Part model, mm, in its own coordinate system. Face numbers are marked on the shaded views. A direction names the side the tool comes from. Coordinates: 2 decimals unless noted, no trailing zeros. Write each loop counter-clockwise with the first axis right and the second up, starting at its lowest first coordinate (ties: lowest second). Pieces come first, ordered by that corner, then holes. Notation, with made-up numbers: (78, 10) -> (83, 10) arc R3 ccw to (83, 15) -> close; hole circle Ø5 at (88.5, 36). An arc over 180 degrees is marked (long way). Write item = value, one per line. Start each with the question number.
Q1. Band-saw the part on C-C, the plane y = 26.5. List the corners of the cut face in (x, z), plus the area to 3 significant figures.
Q2. Band-saw the part on A-A, the plane z = 21. List the corners of the cut face in (x, y), plus the area to 3 significant figures.
Q3. Probe line 1 (Z direction, x = 35.5, y = 18); line 2 (X direction, y = 26, z = 22); line 3 (Y direction, x = 20, z = 18). List the from-to ranges inside material, lowest first.
Q4. Band-saw the part on B-B, the plane x = 14. List the corners of the cut face in (y, z), plus the area to 3 significant figures.
Q5. Pull direction X, two halves, no side cores. Call the marked faces 3, 4, 5 and 6: released by +X, released by -X, zero draft, split by the parting line, or undercut.
Q6. Band-saw the part on D-D, the plane x = 4. List the corners of the cut face in (y, z).
Q7. Pin check, flat tips, straight feed: P1, Ø5, axis at x = 16.5, y = 18, coming from the +Z side; P2, Ø3, axis at x = 37, z = 17.5, coming from the -Y side. Stop position of each tip, or through.
Q8. Tool access for the marked faces 1 and 2: list every direction of +Z, -Z, +X, -X, +Y, -Y with a clear straight run to the whole face (end or side of a thin tool).
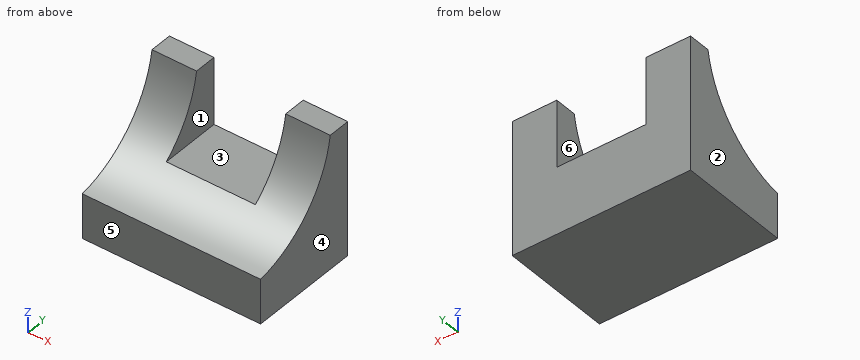
from build123d import *

# Parameters (mm, degrees)
F0_W     = 50.8
F0_H     = 12.7
F1_DEPTH = 31.75
F3_DEPTH = 6.35
F5_DEPTH = 25.4
F7_DEPTH = 50.8
F8_DEPTH = 25.4


with BuildPart() as f1:
    # F0 (on Front) → F1 (new body)
    with BuildSketch(Plane.XZ):
        with Locations((25.4, 6.35)):
            Rectangle(F0_W, F0_H)
    extrude(amount=-F1_DEPTH)

    # F2 (on face) → F3 (join)
    with BuildSketch(Plane(origin=(0, 31.75, 0), x_dir=(-1, 0, 0), z_dir=(0, 1, 0))):
        Polygon((-50.8, 38.1), (-50.8, 12.7), (0, 12.7), (0, 38.1), (-12.7, 38.1), (-12.7, 19.05), (-38.1, 19.05), (-38.1, 38.1), align=None)
    extrude(amount=-F3_DEPTH)

    # F4 (on face) → F5 (join)
    with BuildSketch(Plane.XY.offset(38.1)):
        Polygon((50.8, 0), (50.8, 25.4), (38.1, 25.4), (0, 25.4), (0, 0), align=None)
    extrude(amount=-F5_DEPTH)

    # F6 (on face) → F7 (cut)
    with BuildSketch(Plane.YZ.offset(50.8)):
        with BuildLine():
            Line((0, 38.1), (0, 12.7))
            ThreePointArc((0, 12.7), (16.8424565007, 21.2575434993), (25.4, 38.1))
            Line((25.4, 38.1), (0, 38.1))
        make_face()
    extrude(amount=-F7_DEPTH, mode=Mode.SUBTRACT)

    # F8 (cut): a face of the model
    f8_faces = [f1.faces().sort_by_distance(p)[0] for p in [
        (25.4, 25.4, 28.575),
    ]]
    extrude(f8_faces, amount=-F8_DEPTH, mode=Mode.SUBTRACT)


solid = f1.part
Ans:
q1.outline = (0, 0) -> (50.8, 0) -> (50.8, 38.1) -> (38.1, 38.1) -> (38.1, 19.05) -> (12.7, 19.05) -> (12.7, 38.1) -> (0, 38.1) -> close
q1.area = 1,450 mm2
q2.outline = (0, 16.58) -> (12.7, 16.58) -> (12.7, 31.75) -> (0, 31.75) -> close; (38.1, 16.58) -> (50.8, 16.58) -> (50.8, 31.75) -> (38.1, 31.75) -> close
q2.area = 385 mm2
q3.line_1 = 0 to 19.05
q3.line_2 = 0 to 12.7, 38.1 to 50.8
q3.line_3 = 12.99 to 31.75
q4.outline = (0, 0) -> (31.75, 0) -> (31.75, 19.05) -> (14.38, 19.05) arc R30.46 cw to (0, 12.7) -> close
q4.area = 548 mm2
q5.face_3 = undercut
q5.face_4 = released by +X
q5.face_5 = zero draft
q5.face_6 = undercut
q6.outline = (0, 0) -> (31.75, 0) -> (31.75, 38.1) -> (25.4, 38.1) arc R30.46 cw to (0, 12.7) -> close
q7.P1 = 19.05
q7.P2 = 9.79
q8.face_1 = +Z, +Y, -Y
q8.face_2 = +Z, -Z, -X, +Y, -Y
